```python
from build123d import *

# Parameters (mm, degrees)
SKETCH1_R           = 2.5
BOSS_EXTRUDE1_DEPTH = 3


with BuildPart() as part:
    # Sketch1 → Boss-Extrude1 (new body)
    with BuildSketch(Plane(origin=(0, 0, 0), x_dir=(1, 0, 0), z_dir=(0, 1, 0))):
        Polygon((150, 130.2), (147, 130.2), (147, 157), (120, 157), (120, 160), (90, 160), (90, 157), (60, 157), (60, 160), (30, 160), (30, 157), (3, 157), (3, 130.2), (0, 130.2), (0, 100), (3, 100), (3, 70.2), (0, 70.2), (0, 40), (3, 40), (3, 0), (147, 0), (147, 40), (150, 40), (150, 70.2), (147, 70.2), (147, 100), (150, 100), align=None)
        with Locations((75, 80)):
            Circle(SKETCH1_R, mode=Mode.SUBTRACT)
    extrude(amount=BOSS_EXTRUDE1_DEPTH)


solid = part.part
```
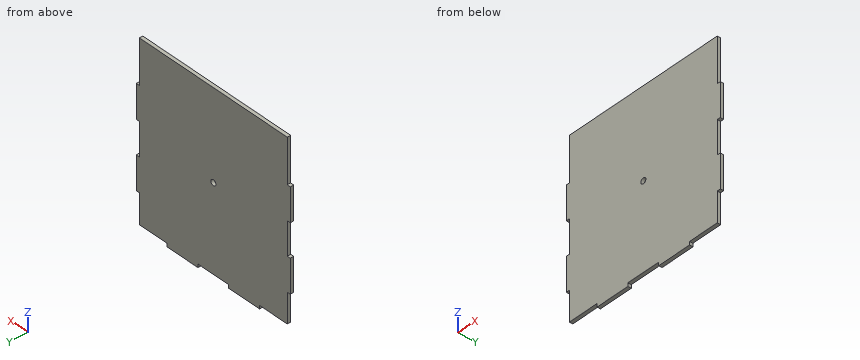
The model under review builds one solid part; all positions refer to its coordinate system, in mm. Round coordinates to 2 decimals unless told otherwise and drop trailing zeros. Order: outer loops, then holes, each group sorted by start corner. A loop starts at its lowest first (then second) coordinate and runs counter-clockwise, first axis right, second up.
Item 1: Add section B-B, the plane z = -80. State the section outline as (x, y) points.
Working result:
outline: (3, 0) - (72.5, 0) - (72.5, 3) - (3, 3) - close; (77.5, 0) - (147, 0) - (147, 3) - (77.5, 3) - close
Item 2: For pin 1 (0.9 mm diameter, centred on y = 2, z = -158, fed in from -X); pin 2 (1.5 mm diameter, centred on y = 2, z = -143.5, fed in from +X); pin 3 (1.5 mm diameter, centred on y = 1, z = -19, fed in from -X), all flat-tipped, find the tip position at first contact; note any pin that passes through.
Working result:
pin 1: stops at x = 30
pin 2: stops at x = 147
pin 3: stops at x = 3
Item 3: To check wall thickness, follow probe 1 along Z at (x, y) = (75, 1.5); probe 2 along X at (y, z) = (0.85, -80); probe 3 along X at (y, z) = (2.55, -94). State the ranges of each line that lie inside material, in increasing order.
Working result:
probe 1: z = -157 to -82.5, -77.5 to 0
probe 2: x = 3 to 72.5, 77.5 to 147
probe 3: x = 3 to 147
Item 4: Add section D-D, the plane z = -147. State the section outline as (x, y) points, and give its area (3 significant figures).
Working result:
outline: (3, 0) - (147, 0) - (147, 3) - (3, 3) - close
area: 432 mm2
Item 5: Add section A-A, the plane x = 75. State the section outline as (y, z) points.
Working result:
outline: (0, -157) - (3, -157) - (3, -82.5) - (0, -82.5) - close; (0, -77.5) - (3, -77.5) - (3, 0) - (0, 0) - close
